Job drawing, mm, ordinate dimensions from the low corner. One solid piece. Give positions to 0.01 mm unless a question says otherwise; leave off trailing zeros. Write each loop counter-clockwise with the first axis right and the second up, starting at its lowest first coordinate (ties: lowest second). Pieces come first, ordered by that corner, then holes. Notation, with made-up numbers: M 48,-9.5 L 72,-9.5 A31 ccw 72,22.5 Z; hole C -3.75,-20 d8. An arc over 180 degrees is marked long. Answer as CSV lines item,"result". Start each with the question number.
1) Slice it at A-A, the plane z = 17.75. Give the cut face in (x, y), plus the area to 3 significant figures.
2) Mould opens along X. For the marked faces 1, 2 and 3 say: pulls with the +X half, pulls with the -X half, needs draft (parallel to the pull), parting line crosses it, or undercut.
3) Wall check: line 1 along Z through (x, y) = (44, 37) (3 decimals); line 2 along Y through (x, z) = (17.5, 18.5). Give the ranges that are in metal, low to high. Write a range as from..to.
4) Slice it at B-B, the plane y = 38.5. Give the cut face in (x, z).
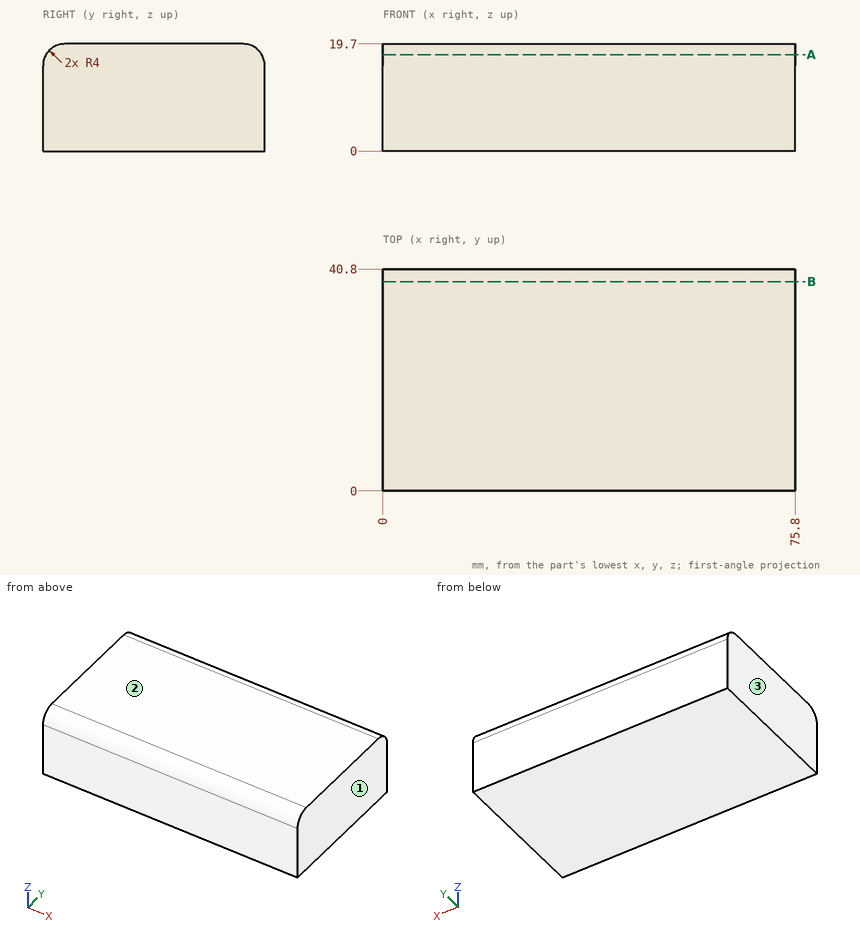
Found:
1,outline,"M 0,0.57 L 75.8,0.57 L 75.8,40.23 L 0,40.23 Z"
1,area,"3,010 mm²"
2,face 1,"pulls with the +X half"
2,face 2,"needs draft"
2,face 3,"pulls with the -X half"
3,line 1,"0..19.695"
3,line 2,"1.14..39.66"
4,outline,"M 0,0 L 75.8,0 L 75.8,19.32 L 0,19.32 Z"
